from build123d import *

# Parameters (mm, degrees)
F0_R     = 3
F2_DEPTH = 8
F3_R     = 10
F4_R     = 5


with BuildPart() as f2:
    # F0 (on Front) → F2 (new body)
    with BuildSketch(Plane.XZ):
        with BuildLine():
            Line((-115, 40), (-150, 40))
            Line((-150, 40), (-150, -40))
            Line((-150, -40), (-125, -40))
            add(Edge.make_bspline(
                [(-125, -40), (-119.8519719708, -11.7183000191), (-120.3236686159, 4.6519688966), (-92.7757024765, 15.9931648523), (-115, 40)],
                knots=[0, 0, 0, 0, 0.5311625984, 1, 1, 1, 1], degree=3))
        make_face()
        with Locations((-140, 10)):
            Circle(F0_R, mode=Mode.SUBTRACT)
        with Locations((-140, 30)):
            Circle(F0_R, mode=Mode.SUBTRACT)
    extrude(amount=F2_DEPTH)

    # F3
    f3_edges = [f2.edges().sort_by_distance(p)[0] for p in [
        (-150, -4, -40),
    ]]
    fillet(f3_edges, radius=F3_R)

    # F4
    f4_edges = [f2.edges().sort_by_distance(p)[0] for p in [
        (-125, -4, -40),
    ]]
    fillet(f4_edges, radius=F4_R)


solid = f2.part
Input: part model. Units: mm. Frame: model coordinates. Give positions to 0.01 mm unless a question says otherwise; leave off trailing zeros. Write each question's results on one line, items separated by ' | '.
Item 1: Section A-A (y = -4.75). Give the number of separate pieces and of enclosed holes in the cut face, and give its area (3 significant figures).
A:
separate pieces: 1 | enclosed holes: 2 | area: 2,770 mm^2
Item 2: Material intervals for line 1 along Z through (x, y) = (-140, -2); line 2 along X through (y, z) = (-4.25, 8.5); line 3 along X through (y, z) = (-5, 5), sorted ascending.
A:
line 1: z = -40 to 7, 13 to 27, 33 to 40 | line 2: x = -150 to -142.6, -137.4 to -107.58 | line 3: x = -150 to -111.63
Item 3: Contact query for a flat-ended pin moving along its axis: pin 1 Ø9.5 at (x, z) = (-140, 10) entering from -Y. Output: stop coordinate, or through.
A:
pin 1: stops at y = -8
Item 4: Draft query along X for faces 1 (the flat face through (-128, 0, 1)), 2 (the cylindrical face through (-147.15, -4.06, -36.99)), 3 (the cylindrical face through (-137.14, -3.94, 30.9)). Return one class per face: released by +X, released by -X, zero draft, split by the parting line, or undercut.
A:
face 1: zero draft | face 2: released by -X | face 3: undercut
